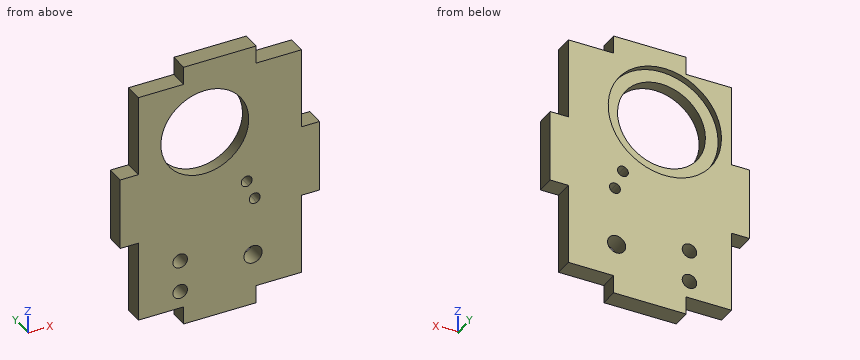
```python
from build123d import *

# Parameters (mm, degrees)
SKETCH1_W           = 90
SKETCH1_H           = 130
SKETCH1_W_2         = 10
SKETCH1_H_2         = 40
SKETCH1_W_3         = 40
SKETCH1_H_3         = 10
BOSS_EXTRUDE1_DEPTH = 10
SKETCH2_R           = 4
CUT_EXTRUDE1_DEPTH  = 173.336879396
CUT_EXTRUDE2_DEPTH  = 173.336879396
SKETCH4_R           = 31.25
CUT_EXTRUDE3_DEPTH  = 3.5
SKETCH5_R           = 24.25
CUT_EXTRUDE4_DEPTH  = 173.169248125
SKETCH6_R           = 5
CUT_EXTRUDE5_DEPTH  = 173.336879396


with BuildPart() as part:
    # Sketch1 → Boss-Extrude1 (new body)
    with BuildSketch(Plane(origin=(0, 0, 0), x_dir=(1, 0, 0), z_dir=(0, 1, 0))):
        with Locations((45, 65)):
            Rectangle(SKETCH1_W, SKETCH1_H)
        with Locations((-5, 65)):
            Rectangle(SKETCH1_W_2, SKETCH1_H_2)
        with Locations((95, 65)):
            Rectangle(SKETCH1_W_2, SKETCH1_H_2)
        with Locations((45, -5)):
            Rectangle(SKETCH1_W_3, SKETCH1_H_3)
        with Locations((45, 135)):
            Rectangle(SKETCH1_W_3, SKETCH1_H_3)
    extrude(amount=BOSS_EXTRUDE1_DEPTH)

    # Sketch2 → Cut-Extrude1 (cut, through all)
    with BuildSketch(Plane(origin=(0, 10, 0), x_dir=(1, 0, 0), z_dir=(0, 1, 0))):
        with Locations(Location((23.122776972, 102.57, 0), (0, 0, 270))):
            Circle(SKETCH2_R)
        with Locations(Location((23.122776972, 120.41, 0), (0, 0, 270))):
            Circle(SKETCH2_R)
    extrude(amount=-CUT_EXTRUDE1_DEPTH, mode=Mode.SUBTRACT)

    # Sketch3 → Cut-Extrude2 (cut, through all)
    with BuildSketch(Plane(origin=(0, 10, 0), x_dir=(1, 0, 0), z_dir=(0, 1, 0))):
        with BuildLine():
            ThreePointArc((65.351977614, 81.42565129), (61.457970709, 79.741397678), (63.142224321, 75.847390774))
            Line((63.142224321, 75.847390774), (65.351977614, 81.42565129))
        make_face()
        with BuildLine():
            Line((65.351977614, 81.42565129), (63.142224321, 75.847390774))
            ThreePointArc((63.142224321, 75.847390774), (65.93312737, 76.155127276), (67.247100967, 78.636521032))
            ThreePointArc((67.247100967, 78.636521032), (66.728494723, 80.322547434), (65.351977614, 81.42565129))
        make_face()
        with BuildLine():
            ThreePointArc((58.722717735, 64.690869742), (61.513620784, 64.998606245), (62.827594381, 67.48))
            Line((62.827594381, 67.48), (59.827594381, 67.48))
            Line((59.827594381, 67.48), (58.722717735, 64.690869742))
        make_face()
        with BuildLine():
            Line((59.827594381, 67.48), (62.827594381, 67.48))
            ThreePointArc((62.827594381, 67.48), (62.308988137, 69.166026403), (60.932471028, 70.269130258))
            Line((60.932471028, 70.269130258), (59.827594381, 67.48))
        make_face()
        with BuildLine():
            Line((58.722717735, 64.690869742), (59.827594381, 67.48))
            Line((59.827594381, 67.48), (56.827594381, 67.48))
            ThreePointArc((56.827594381, 67.48), (57.346200626, 65.793973597), (58.722717735, 64.690869742))
        make_face()
        with BuildLine():
            Line((56.827594381, 67.48), (59.827594381, 67.48))
            Line((59.827594381, 67.48), (60.932471028, 70.269130258))
            ThreePointArc((60.932471028, 70.269130258), (58.141567979, 69.961393755), (56.827594381, 67.48))
        make_face()
    extrude(amount=-CUT_EXTRUDE2_DEPTH, mode=Mode.SUBTRACT)

    # Sketch4 → Cut-Extrude3 (cut)
    with BuildSketch(Plane(origin=(0, 10, 0), x_dir=(1, 0, 0), z_dir=(0, 1, 0))):
        with Locations(Location((36.72, 31.47, 0), (0, 0, 270))):
            Circle(SKETCH4_R)
    extrude(amount=-CUT_EXTRUDE3_DEPTH, mode=Mode.SUBTRACT)

    # Sketch5 → Cut-Extrude4 (cut, through all)
    with BuildSketch(Plane(origin=(0, 6.5, 0), x_dir=(1, 0, 0), z_dir=(0, 1, 0))):
        with Locations(Location((36.72, 31.47, 0), (0, 0, 270))):
            Circle(SKETCH5_R)
    extrude(amount=-CUT_EXTRUDE4_DEPTH, mode=Mode.SUBTRACT)

    # Sketch6 → Cut-Extrude5 (cut, through all)
    with BuildSketch(Plane(origin=(0, 10, 0), x_dir=(1, 0, 0), z_dir=(0, 1, 0))):
        with Locations(Location((63.314917683, 111.209559188, 0), (0, 0, 270))):
            Circle(SKETCH6_R)
    extrude(amount=-CUT_EXTRUDE5_DEPTH, mode=Mode.SUBTRACT)


solid = part.part
```
Geometry check sheet. Reference: the model listing, model coordinates, mm. Coordinates: 2 decimals unless noted, no trailing zeros. Loops run counter-clockwise (first coordinate to the right, second up) from the corner with the lowest first, then second, coordinate; pieces in that order, holes last. Notation, with made-up numbers: (-29, 26.5) -> (12, 26.5) arc R29 ccw to (12, 65.5) -> close; hole circle Ø2 at (73, 13). An arc over 180 degrees is marked (long way). Put each result on its own line as item: value.
1) Thickness scan on line 1 (X direction, y = 5.75, z = -102.57); line 2 (Z direction, x = 1, y = 1); line 3 (X direction, y = 3, z = -23.5). Record the ranges inside material, lowest first.
Result set:
line 1: x = 0 to 19.12, 27.12 to 90
line 2: z = -130 to 0
line 3: x = 0 to 13.82, 59.62 to 90
2) Gauge pin test, flat ends, axial feed: pin 1 Ø5 at (y, z) = (2.5, 3) entering from -X; pin 2 Ø3 at (x, y) = (76.5, 6.5) entering from +Z; pin 3 Ø3 at (y, z) = (6.5, 3) entering from +X. Record the tip position at first contact, or that the pin passes through.
Result set:
pin 1: stops at x = 25
pin 2: stops at z = 0
pin 3: stops at x = 65
3) Cross-section at C-C on z = -102.57. Record the boundary of the cut face in (x, y), plus the area to 3 significant figures.
Result set:
outline: (0, 0) -> (19.12, 0) -> (19.12, 10) -> (0, 10) -> close; (27.12, 0) -> (90, 0) -> (90, 10) -> (27.12, 10) -> close
area: 820 mm^2
4) Cross-section at B-B on z = -31.47. Record the boundary of the cut face in (x, y).
Result set:
outline: (0, 0) -> (12.47, 0) -> (12.47, 6.5) -> (5.47, 6.5) -> (5.47, 10) -> (0, 10) -> close; (60.97, 0) -> (90, 0) -> (90, 10) -> (67.97, 10) -> (67.97, 6.5) -> (60.97, 6.5) -> close
5) Cross-section at D-D on x = 76.5. Record the boundary of the cut face in (y, z), plus the area to 3 significant figures.
Result set:
outline: (0, -130) -> (10, -130) -> (10, 0) -> (0, 0) -> close
area: 1,300 mm^2
6) Cross-section at A-A on x = 36.72. Record the boundary of the cut face in (y, z).
Result set:
outline: (0, -140) -> (10, -140) -> (10, -62.72) -> (6.5, -62.72) -> (6.5, -55.72) -> (0, -55.72) -> close; (0, -7.22) -> (6.5, -7.22) -> (6.5, -0.22) -> (10, -0.22) -> (10, 10) -> (0, 10) -> close
